Autodesk Inventor part; units mm, degrees
ref_plane "YZ Plane" through (0, 0, 0) normal (1, 0, 0) x (0, 1, 0)
ref_plane "XZ Plane" through (0, 0, 0) normal (0, 1, 0) x (-1, 0, 0)
ref_plane "XY Plane" through (0, 0, 0) normal (0, 0, 1) x (1, 0, 0)
sketch "Sketch1" plane through (0, 0, 0) normal (0, 0, 1) x (1, 0, 0)
  line L0 (0, 0) -> (34.5, 0)
  line L1 (34.5, 0) -> (34.5, 54)
  line L2 (34.5, 54) -> (0, 54)
  line L3 (0, 54) -> (0, 0)
  dimension "d0" = 54
  dimension "d1" = 34.5
extrude "Extrusion1" add sketch "Sketch1" along normal blind 12.25
sketch "Sketch2" plane through (0, 0, 12.25) normal (0, 0, 1) x (1, 0, 0)
  line L0 (12.25, 41) -> (17.25, 49.6603)
  line L1 (17.25, 49.6603) -> (22.25, 41)
  line L2 (22.25, 41) -> (12.25, 41)
  line L3 (0, 0) -> (34.5, 0) construction
  point P0 (17.25, 41)
  point P1 (17.25, 0)
  dimension "d4" = 41
  dimension "d5" = 10
extrude "Extrusion2" cut sketch "Sketch2" against normal blind 0.1
sketch "Sketch3" plane through (0, 54, 0) normal (0, 1, 0) x (1, 0, 0)
  line L0 (34.5, 0) -> (0, 0) construction
  line L1 (0, 0) -> (0, -12.25) construction
  line L2 (34.5, -12.25) -> (0, -12.25) construction
  line L3 (34.5, 0) -> (34.5, -12.25) construction
  line L4 (4, 0) -> (4, -3)
  line L5 (4, -3) -> (0, -3)
  line L6 (4, 0) -> (0, 0)
  line L7 (0, -3) -> (0, 0)
  point P0 (0, 0)
  dimension "d8" = 3
  dimension "d9" = 4
extrude "Extrusion3" cut sketch "Sketch3" against normal blind 3
sketch "Sketch4" plane through (0, 54, 12.25) normal (0, 1, 0) x (1, 0, 0)
  line L0 (4, 12.25) -> (4, 9.25)
  line L1 (4, 9.25) -> (0, 9.25)
  line L2 (0, 9.25) -> (0, 0)
  line L3 (34.5, 0) -> (0, 0)
  line L4 (34.5, 12.25) -> (34.5, 0)
  line L5 (34.5, 12.25) -> (4, 12.25)
  line L6 (6, 10.1) -> (10, 10.1)
  line L7 (10, 10.1) -> (10, 5.2)
  line L8 (10, 5.2) -> (6, 5.2)
  line L9 (6, 5.2) -> (6, 10.1)
  line L10 (12.6, 10.1) -> (16.6, 10.1)
  line L11 (16.6, 10.1) -> (16.6, 5.2)
  line L12 (16.6, 5.2) -> (12.6, 5.2)
  line L13 (12.6, 5.2) -> (12.6, 10.1)
  line L14 (19.2, 10.1) -> (23.2, 10.1)
  line L15 (23.2, 10.1) -> (23.2, 5.2)
  line L16 (23.2, 5.2) -> (19.2, 5.2)
  line L17 (19.2, 5.2) -> (19.2, 10.1)
  line L18 (10, 10.1) -> (12.6, 10.1) construction
  line L19 (2, 4.16) -> (4.43, 4.16)
  line L20 (4.43, 4.16) -> (4.43, 8.8603)
  line L21 (4.43, 8.8603) -> (2, 8.8603)
  line L22 (2, 8.8603) -> (2, 4.16)
  point P0 (0, 12.25)
  dimension "d12" = 2.15
  dimension "d13" = 4.9
  dimension "d14" = 6
  dimension "d15" = 4
  dimension "d16" = 12.6
  dimension "d17" = 2.6
  dimension "d18" = 2.6
  dimension "d21" = 2
  dimension "d22" = 4.7003
  dimension "d23" = 2.43
  dimension "d24" = 4.16
extrude "Extrusion4" cut sketch "Sketch4" against normal blind 0.9 contours L6 L7 L8 L9 | L10 L11 L12 L13 | L14 L15 L16 L17
sketch "Sketch5" plane through (0, 54, 12.25) normal (0, 1, 0) x (1, 0, 0)
  line L0 (20.3264, 2.5717) -> (22.0736, 2.5717) construction
  line L1 (22.0736, 2.5717) -> (22.0736, 2.1463) construction
  line L2 (22.0736, 2.1463) -> (20.3264, 2.1463) construction
  line L3 (20.3264, 2.1463) -> (20.3264, 2.5717) construction
  line L4 (23.2, 5.2) -> (19.2, 5.2)
  line L5 (15.4736, 2.1463) -> (13.7264, 2.1463) construction
  line L6 (13.7264, 2.1463) -> (13.7264, 2.5717) construction
  line L7 (13.7264, 2.5717) -> (15.4736, 2.5717) construction
  line L8 (15.4736, 2.5717) -> (15.4736, 2.1463) construction
  line L9 (16.6, 5.2) -> (12.6, 5.2)
  line L10 (8.8736, 2.5717) -> (8.8736, 2.1463) construction
  line L11 (8.8736, 2.1463) -> (7.1264, 2.1463) construction
  line L12 (7.1264, 2.1463) -> (7.1264, 2.5717) construction
  line L13 (7.1264, 2.5717) -> (8.8736, 2.5717) construction
  line L14 (10, 5.2) -> (6, 5.2)
  point P0 (0, 12.25)
  point P1 (21.2, 5.2)
  point P2 (21.2, 2.5717)
  point P3 (14.6, 2.1463)
  point P4 (14.6, 5.2)
  point P5 (8, 2.1463)
  point P6 (8, 5.2)
  point P7 (20.3264, 2.359)
  point P8 (15.4736, 2.359)
  point P9 (8.8736, 2.359)
  dimension "d25" = 2.6283
  dimension "d26" = 1.7472
  dimension "d27" = 0.4254
equation "\"d18\" = d17"
properties part number "battery model"
CAD build for the part. Positions are in the model's coordinates, mm. A direction names the side the tool comes from. Give positions to 0.01 mm unless a question says otherwise; leave off trailing zeros. Put each result on its own line as item: value.
(1) Tool access for faces 4 (the flat face through (21, 53.1, 5)), 5 (the flat face through (34.5, 27, 6)), 6 (the flat face through (2, 51, 1)): list every direction of +Z, -Z, +X, -X, +Y, -Y with a clear straight run to the whole face (end or side of a thin tool).
Working result:
face 4: +Y
face 5: +Z, -Z, +X, +Y, -Y
face 6: -Z, -X, +Y
(2) Wall check: L1, parallel to Y at x = 16.5, z = 4. Give the ranges that are in metal, low to high.
Working result:
L1: 0 to 53.1
(3) Pull direction Z, two halves, no side cores. Call faces 1 (the flat face through (17, 27, 0)), 2 (the flat face through (17, 44, 12.15)), 3 (the flat face through (8, 53.1, 5)): released by +Z, released by -Z, zero draft, split by the parting line, or undercut.
Working result:
face 1: released by -Z
face 2: released by +Z
face 3: undercut
(4) Drop flat-ended pins along their axis: pin 1 Ø1.5 at (x, z) = (1.5, 2) entering from +Y; pin 2 Ø1.2 at (x, z) = (7.5, 4.5) entering from +Y; pin 3 Ø3.5 at (x, y) = (2, 53) entering from -Z. Give the stop position or say it passes through.
Working result:
pin 1: y = 51
pin 2: y = 53.1
pin 3: z = 3
